Geometry: see drawing. Coordinates: mm, zero at the bounding-box minimum. Round coordinates to 2 decimals unless told otherwise and drop trailing zeros. Loops run counter-clockwise (first coordinate to the right, second up) from the corner with the lowest first, then second, coordinate; pieces in that order, holes last.
(1) First-contact query: pin 1 Ø6.5 at (x, y) = (131.19, 31.75) entering from +Z; pin 2 Ø3 at (x, z) = (47.5, 16) entering from +Y; pin 3 Ø6 at (y, z) = (11, 16) entering from +X; pin 4 Ø1.5 at (y, z) = (10.5, 6.5) entering from +X. Flat tips, straight axial feed; report the tip coordinate or a pass-through.
(2) Draft query along X for the marked faces 1, 2 and 3. Return one class per face: released by +X, released by -X, zero draft, split by the parting line, or undercut.
(3) Cut plane D-D, the plane z = 12.5. Output: boundary loops of the cut face in (x, y), and give its area (3 significant figures).
(4) Cut plane B-B, the plane y = 31.75. Give the number of separate pieces and of enclosed holes in the cut face, and give its area (3 significant figures).
(5) Line query: line 1 (Y direction, x = 76.2, z = 11); line 2 (Z direction, x = 97, y = 57.5); line 3 (Y direction, x = 106, z = 11) (1 decimal). Output: solid intervals per line, ascending.
(6) Cut plane A-A, the plane x = 76.2. Output: boundary loops of the cut face in (y, z), and give its area (3 significant figures).
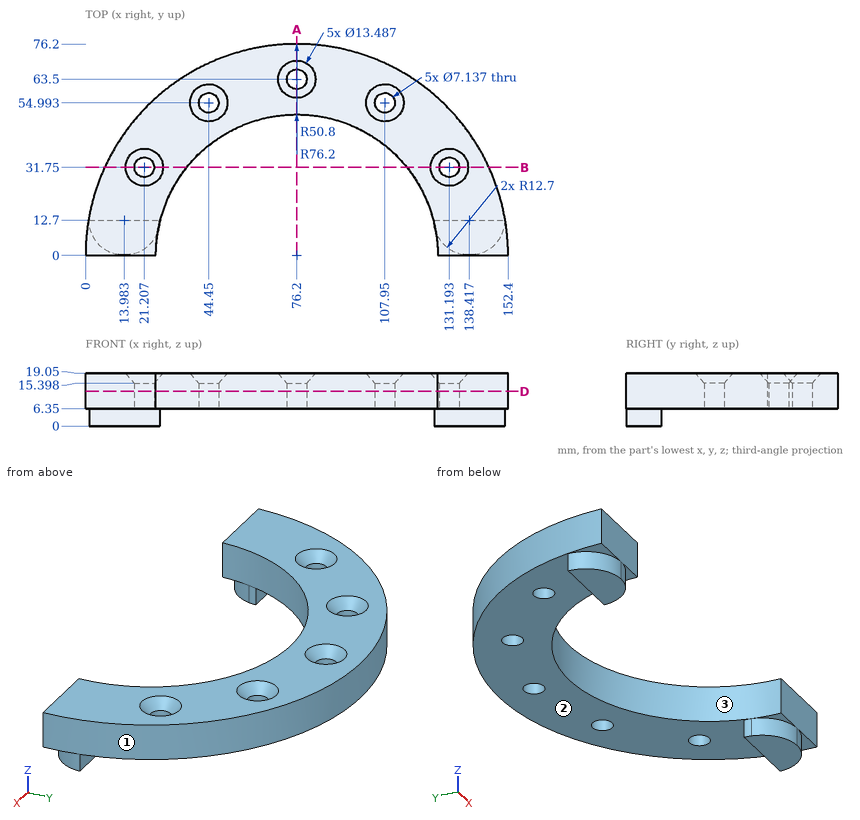
Reported:
1. pin 1: passes through
1. pin 2: stops at y = 71.18
1. pin 3: stops at x = 151.98
1. pin 4: stops at x = 151.77
2. face 1: split by the parting line
2. face 2: zero draft
2. face 3: undercut
3. outline: (0, 0) - (25.4, 0) arc R50.8 cw to (127, 0) - (152.4, 0) arc R76.2 ccw to start; hole circle Ø7.14 at (21.21, 31.75); hole circle Ø7.14 at (44.45, 54.99); hole circle Ø7.14 at (76.2, 63.5); hole circle Ø7.14 at (107.95, 54.99); hole circle Ø7.14 at (131.19, 31.75)
3. area: 4,870 mm2
4. separate pieces: 4
4. enclosed holes: 0
4. area: 548 mm2
5. line 1: y = 50.8 to 59.93, 67.07 to 76.2
5. line 2: z = 6.35 to 19.05
5. line 3: y = 41.1 to 52, 58 to 70.1
6. outline: (50.8, 6.35) - (59.93, 6.35) - (59.93, 15.4) - (56.76, 19.05) - (50.8, 19.05) - close; (67.07, 6.35) - (76.2, 6.35) - (76.2, 19.05) - (70.24, 19.05) - (67.07, 15.4) - close
6. area: 220 mm2
